Verification items for the finished model (mm, model axes). A direction names the side the tool comes from. Coordinates: 2 decimals unless noted, no trailing zeros. Order: outer loops, then holes, each group sorted by start corner. A loop starts at its lowest first (then second) coordinate and runs counter-clockwise, first axis right, second up. Notation, with made-up numbers: M 43.5,29.5 L 97.5,29.5 A22 ccw 97.5,43.5 Z; hole C 43,-35 d3. An arc over 180 degrees is marked long. Return JSON: item names as keys, results as strings. Group by question number.
Q1. Go/stop test with flat-tipped pins: pin 1 Ø2 at (x, z) = (2.5, -0.5) entering from -Y; pin 2 Ø0.9 at (y, z) = (2.5, -1.5) entering from +X. Record where each tip stops, or that it passes through.
Q2. Section check A-A, the plane y = 2.4. Enter the section's corners in (x, z), then the cut area to 3 significant figures.
Q3. Section check B-B, the plane z = -2.35. Enter the section's corners in (x, y).
Q4. Mould release check, pull along X, two halves, no side actions. Record for faces 5 (the face through (3, 2, 1)), 6 (the face through (1, 3, 1)), 7 (the face through (-2, 2, 0)): pulls with the +X half, pulls with the -X half, needs draft (parallel to the pull), parting line crosses it, or undercut.
Q5. Section check D-D, the plane x = -0.15. Enter the section's corners in (y, z), then the cut area to 3 significant figures.
Q6. Thickness scan on probe 1 along X at (y, z) = (2.8, 0.5); probe 2 along X at (y, z) = (1.55, -2.4); probe 3 along Y at (x, z) = (1.7, 0.6). Record the ranges inside material, lowest first.
Q7. Section check C-C, the plane y = 0.55. Enter the section's corners in (x, z) (3 decimals).
Q8. Access from +Z, -Z, +X, -X, +Y, -Y to the whole of each face (thin tool, end or side, straight path). Record for faces 1 (the face through (-2, 2, -3)), 2 (the face through (0, 2, 0)), 3 (the face through (2, 2.5, 0)), 4 (the face through (-1, 2, 2)).
from build123d import *

# Parameters (mm, degrees)
SKETCH1_W           = 6
SKETCH1_H           = 6
BOSS_EXTRUDE1_DEPTH = 5
CUT_EXTRUDE1_DEPTH  = 2
CUT_EXTRUDE2_DEPTH  = 2
CUT_EXTRUDE3_DEPTH  = 2


with BuildPart() as part:
    # Sketch1 → Boss-Extrude1 (new body)
    with BuildSketch(Plane(origin=(0, 0, 0), x_dir=(1, 0, 0), z_dir=(0, 1, 0))):
        Rectangle(SKETCH1_W, SKETCH1_H)
    extrude(amount=BOSS_EXTRUDE1_DEPTH)

    # Sketch2 → Cut-Extrude1 (cut)
    with BuildSketch(Plane.ZY.offset(3)):
        Polygon((3, 5), (-3, 5), (-3, 4), (3, 0), align=None)
    extrude(amount=-CUT_EXTRUDE1_DEPTH, mode=Mode.SUBTRACT)

    # Sketch3 → Cut-Extrude2 (cut)
    with BuildSketch(Plane.ZY.offset(1)):
        Polygon((-3, 0), (3, 4), (3, 5), (-3, 5), align=None)
    extrude(amount=-CUT_EXTRUDE2_DEPTH, mode=Mode.SUBTRACT)

    # Sketch4 → Cut-Extrude3 (cut)
    with BuildSketch(Plane.ZY.offset(-1)):
        Polygon((-3, 0), (3, 5), (-3, 5), align=None)
    extrude(amount=-CUT_EXTRUDE3_DEPTH, mode=Mode.SUBTRACT)


solid = part.part
Numbers:
{
 "1": {"pin 1": "stops at y = 0", "pin 2": "stops at x = -1"},
 "2": {"outline": "M -3,-3 L -1,-3 L -1,-0.6 L -3,-0.6 Z; M -1,0.6 L 1,0.6 L 1,-0.12 L 3,-0.12 L 3,3 L -1,3 Z", "area": "15.8 mm2"},
 "3": {"outline": "M -3,0 L 3,0 L 3,0.54 L 1,0.54 L 1,0.43 L -1,0.43 L -1,3.57 L -3,3.57 Z"},
 "4": {"face 5": "pulls with the +X half", "face 6": "undercut", "face 7": "needs draft"},
 "5": {"outline": "M 0,-3 L 4,3 L 0,3 Z", "area": "12.0 mm2"},
 "6": {"probe 1": "x = 1 to 3", "probe 2": "x = -3 to -1", "probe 3": "y = 0 to 3"},
 "7": {"outline": "M -3,-3 L -1,-3 L -1,-2.175 L 1,-2.175 L 1,-2.34 L 3,-2.34 L 3,3 L -1,3 L -1,2.175 L -3,2.175 Z"},
 "8": {"face 1": "-Z, +X, -X, +Y, -Y", "face 2": "-Z, +Y", "face 3": "-Z, +X, +Y", "face 4": "+Z, -X, +Y"}
}
